The drawing under review shows one solid part. Ordinate dimensions are in mm from its lowest x, y, z. A direction names the side the tool comes from. Coordinates: 2 decimals unless noted, no trailing zeros. Write each loop counter-clockwise with the first axis right and the second up, starting at its lowest first coordinate (ties: lowest second). Pieces come first, ordered by that corner, then holes. Notation, with made-up numbers: M 27.25,-12 L 53.25,-12 A26 cw 53.25,23 Z; hole C -22.75,38.25 d10. An arc over 180 degrees is marked long. Write item = value, one per line.
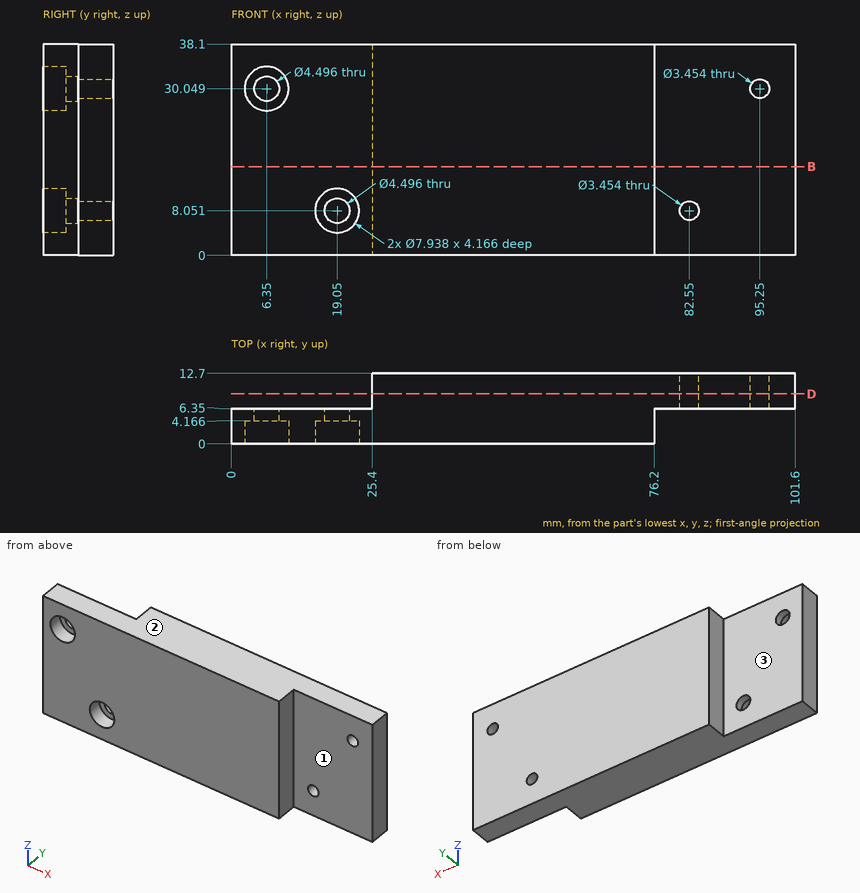
Q1. Machinability: for the marked faces 1, 2 and 3, which of the approach directions +Z, -Z, +X, -X, +Y, -Y give a long, thin tool a straight path to every point of the face, cutting with its end or side? Answer none if there is none.
Check result:
face_1 = +Z, -Z, +X, -Y
face_2 = +Z, +X, -X, +Y, -Y
face_3 = +Z, -Z, -X, +Y
Q2. Consider section D-D, the plane y = 9. State how many separate pieces and enclosed holes the cut face has, and give its area (3 significant figures).
Check result:
separate_pieces = 1
enclosed_holes = 2
area = 2,880 mm²
Q3. For P1, Ø7, axis at x = 19.05, z = 8.05, coming from the -Y side; P2, Ø1.5, axis at x = 37.5, y = 2, coming from the -Z side; P3, Ø5, axis at y = 2, z = 23.5, coming from the +X side; P4, Ø3.5, axis at x = 6.35, z = 30.05, coming from the -Y side, all flat-tipped, find the tip position at first contact; note any pin that passes through.
Check result:
P1 = 4.17
P2 = 0
P3 = 76.2
P4 = through
Q4. Wall thickness on line 1 (Z direction, x = 19.05, y = 2.25); line 2 (Z direction, x = 6.35, y = 1.8); line 3 (Y direction, x = 89.5, z = 9.5): over which ranges is each line inside the solid? List them lowest first.
Check result:
line_1 = 0 to 4.08, 12.02 to 38.1
line_2 = 0 to 26.08, 34.02 to 38.1
line_3 = 6.35 to 12.7
Q5. Consider section B-B, the plane z = 16. State the section outline as (x, y) points.
Check result:
outline = M 0,0 L 76.2,0 L 76.2,6.35 L 101.6,6.35 L 101.6,12.7 L 25.4,12.7 L 25.4,6.35 L 0,6.35 Z
